For this review, take the finished solid that the model builds, in its own axes (mm). A direction names the side the tool comes from. Coordinates: 2 decimals unless noted, no trailing zeros. Loops run counter-clockwise (first coordinate to the right, second up) from the corner with the lowest first, then second, coordinate; pieces in that order, holes last. Notation, with made-up numbers: M 85,6 L 117,6 A28 cw 117,39 Z; hole C 67,26.25 d8. An arc over 180 degrees is marked long. Put each result on its own line as item: value.
```python
from build123d import *

# Parameters (mm, degrees)
BOSS_EXTRUDE1_DEPTH      = 127
BOSS_EXTRUDE1_DEPTH_BACK = 127
SKETCH1_R                = 10
SKETCH2_R                = 10
SKETCH2_R_2              = 5
BOSS_EXTRUDE2_DEPTH      = 20
BOSS_EXTRUDE3_START      = 20
SKETCH3_R                = 10
SKETCH3_R_2              = 5
BOSS_EXTRUDE3_DEPTH      = 20


with BuildPart() as part:
    # Sketch1 → Boss-Extrude1 (new, two sides: drawn at the far end of the back side and taken through both)
    with BuildSketch(Plane(origin=(0, 0, 0), x_dir=(0, 0, -1), z_dir=(1, 0, 0)).offset(-BOSS_EXTRUDE1_DEPTH_BACK)):
        Circle(SKETCH1_R)
    extrude(amount=BOSS_EXTRUDE1_DEPTH + BOSS_EXTRUDE1_DEPTH_BACK)

    # Sketch2 → Boss-Extrude2 (add)
    with BuildSketch(Plane(origin=(127, 0, 0), x_dir=(0, 0, -1), z_dir=(1, 0, 0))):
        Circle(SKETCH2_R)
        Circle(SKETCH2_R_2, mode=Mode.SUBTRACT)
    extrude(amount=BOSS_EXTRUDE2_DEPTH)

    # Sketch3 → Boss-Extrude3 (add)
    with BuildSketch(Plane.ZY.offset(127).offset(BOSS_EXTRUDE3_START)):
        with Locations(Location((0, 0, 0), (0, 0, 180))):
            Circle(SKETCH3_R)
        with Locations(Location((0, 0, 0), (0, 0, 180))):
            Circle(SKETCH3_R_2, mode=Mode.SUBTRACT)
    extrude(amount=-BOSS_EXTRUDE3_DEPTH)


solid = part.part
```
(1) For pin 1 (2 mm diameter, centred on x = -23, y = 5, fed in from +Z); pin 2 (2 mm diameter, centred on x = 14, z = 3.5, fed in from +Y); pin 3 (3 mm diameter, centred on y = 0, z = -0.5, fed in from -X), all flat-tipped, find the tip position at first contact; note any pin that passes through.
Determined:
pin 1: stops at z = 9.17
pin 2: stops at y = 9.68
pin 3: stops at x = -127
(2) Add section C-C (x = 39.5). Write out the cut boundary in (y, z).
Determined:
outline: C 0,0 d20
(3) Wall thickness on line 1 along Y through (x, z) = (-141, 0); line 2 along X through (y, z) = (-2, -2); line 3 along Y through (x, z) = (31, -1): over which ranges is each line inside the solid? List them lowest first. Write a range as [from, to].
Determined:
line 1: y = [-10, -5], [5, 10]
line 2: x = [-127, 127]
line 3: y = [-9.95, 9.95]
(4) Tool access review of faces 1 (the flat face through (147, -2, 5)), 2 (the flat face through (-127, 0, 0)): name each direction out of +Z, -Z, +X, -X, +Y, -Y from which nothing blocks a thin tool from reaching the whole face with its end or side.
Determined:
face 1: +Z, -Z, +X, +Y, -Y
face 2: -X
(5) Add section A-A (z = 0). Write out the cut boundary in (x, y), plus the area to 3 significant figures.
Determined:
outline: M -147,-10 L 147,-10 L 147,-5 L 127,-5 L 127,5 L 147,5 L 147,10 L -147,10 L -147,5 L -127,5 L -127,-5 L -147,-5 Z
area: 5,480 mm^2
(6) Draft analysis for pull direction Y (two halves, no side actions). For faces 3 (the cylindrical face through (-2, 0, 10)), 4 (the flat face through (127, 0, 0)), 5 (the cylindrical face through (136.86, -4.88, 1.08)), 6 (the flat face through (-147, -5, -2)), state which applies: +Y half, -Y half, draft (parallel to the pull), parting line (faces both ways), or undercut.
Determined:
face 3: parting line
face 4: undercut
face 5: undercut
face 6: draft
